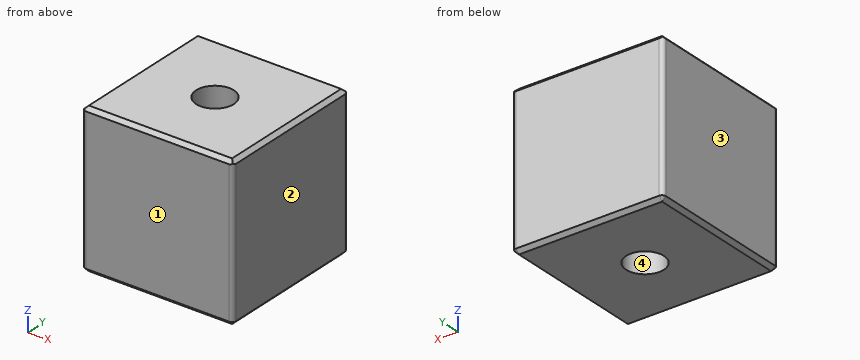
from build123d import *

# Parameters (mm, degrees)
F0_W     = 100
F0_H     = 100
F1_DEPTH = 50
F2_SIZE  = 2.5
F3_R     = 2.5
F4_SIZE  = 2.5
F5_R     = 12.5
F6_DEPTH = 100.001


with BuildPart() as f1:
    # F0 (on Front) → F1 (new body, symmetric)
    with BuildSketch(Plane.XZ):
        Rectangle(F0_W, F0_H)
    extrude(amount=F1_DEPTH, both=True)

    # F2
    f2_edges = [f1.edges().sort_by_distance(p)[0] for p in [
        (50, 0, 50),
        (0, -50, 50),
        (-50, 0, 50),
        (0, 50, 50),
    ]]
    chamfer(f2_edges, length=F2_SIZE)

    # F3
    f3_edges = [f1.edges().sort_by_distance(p)[0] for p in [
        (-50, 50, -1.25),
        (50, -50, -1.25),
        (-50, -50, -1.25),
        (50, 50, -1.25),
    ]]
    fillet(f3_edges, radius=F3_R)

    # F4
    f4_edges = [f1.edges().sort_by_distance(p)[0] for p in [
        (0, -50, -50),
        (0, 50, -50),
        (-50, 0, -50),
        (50, 0, -50),
    ]]
    chamfer(f4_edges, length=F4_SIZE)

    # F5 (on face) → F6 (cut, through all)
    with BuildSketch(Plane(origin=(0, 0, -50), x_dir=(1, 0, 0), z_dir=(0, 0, -1))):
        Circle(F5_R)
    extrude(amount=-F6_DEPTH, mode=Mode.SUBTRACT)


solid = f1.part
Check sheet for the modelled part. Datum: model origin and axes. Units: mm. Face numbers are marked on the shaded views. Give positions to 0.01 mm unless a question says otherwise; leave off trailing zeros. Loops run counter-clockwise (first coordinate to the right, second up) from the corner with the lowest first, then second, coordinate; pieces in that order, holes last. Notation, with made-up numbers: M -4.75,32.5 L 0.25,32.5 A21 cw 0.25,55.5 Z; hole C -33.5,61.5 d4. An arc over 180 degrees is marked long. Return JSON: item names as keys, results as strings. Group by question number.
1. Mould release check, pull along X, two halves, no side actions. Record for the marked faces 1, 2, 3 and 4: released by +X, released by -X, zero draft, split by the parting line, or undercut.
2. Thickness scan on L1, parallel to Y at x = 0, z = 16. Record the ranges inside material, lowest first.
3. Cross-section at A-A on y = 0. Record the boundary of the cut face in (x, z).
4. Cross-section at C-C on z = -4.5. Record the boundary of the cut face in (x, y).
Return value:
{
 "1": {"face 1": "zero draft", "face 2": "released by +X", "face 3": "released by -X", "face 4": "undercut"},
 "2": {"L1": "-50 to -12.5, 12.5 to 50"},
 "3": {"outline": "M -50,-47.5 L -47.5,-50 L -12.5,-50 L -12.5,50 L -47.5,50 L -50,47.5 Z; M 12.5,-50 L 47.5,-50 L 50,-47.5 L 50,47.5 L 47.5,50 L 12.5,50 Z"},
 "4": {"outline": "M -50,-47.5 A2.5 ccw -47.5,-50 L 47.5,-50 A2.5 ccw 50,-47.5 L 50,47.5 A2.5 ccw 47.5,50 L -47.5,50 A2.5 ccw -50,47.5 Z; hole C 0,0 d25"}
}
